Source: CAD feature listing. Evaluate the final solid. Frame: model axes, mm. Face numbers are marked on the shaded views. A direction names the side the tool comes from. Round coordinates to 2 decimals unless told otherwise and drop trailing zeros. Write each loop counter-clockwise with the first axis right and the second up, starting at its lowest first coordinate (ties: lowest second). Pieces come first, ordered by that corner, then holes.
from build123d import *

# Parameters (mm, degrees)
SKETCH1_R                     = 7
BOSS_EXTRUDE1_DEPTH           = 15
BOSS_EXTRUDE1_TAPER           = 3
BOSS_EXTRUDE1_OTHER_WAY_DEPTH = 6
BOSS_EXTRUDE1_OTHER_WAY_TAPER = -3
CUT_EXTRUDE1_DEPTH            = 19.220929184
CUT_EXTRUDE1_DEPTH_BACK       = 19.220929184
CUT_EXTRUDE2_START            = -9.200504543
CUT_EXTRUDE2_OUTLINE_W        = 6.502745185
CUT_EXTRUDE2_OUTLINE_H        = 6
CUT_EXTRUDE2_DEPTH            = 9.200504543
SKETCH5_R                     = 1.5
CUT_EXTRUDE3_DEPTH            = 21.554832283
FILLET1_SIZE                  = 5
CUT_EXTRUDE4_DEPTH            = 19.096992379
CUT_EXTRUDE4_DEPTH_BACK       = 19.096992379
SKETCH6_W                     = 14.909790155
SKETCH6_H                     = 10.479187812
CUT_EXTRUDE5_DEPTH            = 16.143532008


with BuildPart() as part:
    # Sketch1 → Boss-Extrude1 (new body)
    with BuildSketch(Plane(origin=(0, 0, 0), x_dir=(1, 0, 0), z_dir=(0, 1, 0))):
        Circle(SKETCH1_R)
    extrude(amount=BOSS_EXTRUDE1_DEPTH, taper=BOSS_EXTRUDE1_TAPER)

    # Sketch1 → Boss-Extrude1 other way (add)
    with BuildSketch(Plane(origin=(0, 0, 0), x_dir=(1, 0, 0), z_dir=(0, 1, 0))):
        Circle(SKETCH1_R)
    extrude(amount=-BOSS_EXTRUDE1_OTHER_WAY_DEPTH, taper=BOSS_EXTRUDE1_OTHER_WAY_TAPER)

    # Sketch3 → Cut-Extrude1 (cut, two sides: drawn at the far end of the back side and taken through both)
    with BuildSketch(Plane(origin=(0, 0, 0), x_dir=(0, 0, -1), z_dir=(1, 0, 0)).offset(-CUT_EXTRUDE1_DEPTH_BACK)):
        Polygon((-1.886057768, -6), (-1.886057768, 0), (-9.929766736, 8.043708969), (-9.929766736, -6), align=None)
    extrude(amount=CUT_EXTRUDE1_DEPTH + CUT_EXTRUDE1_DEPTH_BACK, mode=Mode.SUBTRACT)

    # Cut-Extrude2: read off the stored shape, not the designer's step
    # Cut-Extrude2 outline → Cut-Extrude2 (cut)
    with BuildSketch(Plane.XY.offset(1.886057768).offset(CUT_EXTRUDE2_START)):
        with Locations((-8.251372593, -3)):
            Rectangle(CUT_EXTRUDE2_OUTLINE_W, CUT_EXTRUDE2_OUTLINE_H)
        with Locations((8.251372593, -3)):
            Rectangle(CUT_EXTRUDE2_OUTLINE_W, CUT_EXTRUDE2_OUTLINE_H)
    extrude(amount=CUT_EXTRUDE2_DEPTH, mode=Mode.SUBTRACT)

    # Sketch5 → Cut-Extrude3 (cut, through all)
    with BuildSketch(Plane(origin=(5, 0, 0), x_dir=(0, 0, -1), z_dir=(1, 0, 0))):
        with Locations((0.613942232, -3.5)):
            Circle(SKETCH5_R)
    extrude(amount=-CUT_EXTRUDE3_DEPTH, mode=Mode.SUBTRACT)

    # Fillet1
    # a fillet whose section is not a circle: 5 mm, written as the material it takes off along each edge
    with BuildSketch(Plane(origin=(17.5, -6, 1.886057768), x_dir=(0, 0, -1), z_dir=(-1, 0, 0))) as fillet1_piece_1:
        with BuildLine():
            Bezier((FILLET1_SIZE, 0), (0, 0), (0, -FILLET1_SIZE), weights=[1, 1.5, 1])
            Line((0, -FILLET1_SIZE), (0, 0))
            Line((0, 0), (FILLET1_SIZE, 0))
        make_face()
    extrude(amount=35, mode=Mode.SUBTRACT)

    # Fillet2
    # a fillet whose section is not a circle: 10, 5 mm, written as the material it takes off along each edge
    with BuildSketch(Plane(origin=(0, 15, 0), x_dir=(1, 0, 0), z_dir=(0, 0, -1))) as fillet2_piece_1:
        with BuildLine():
            Bezier((6.724247047, 9.738320219), (6.213883311, 0), (1.731099374, 0), weights=[1, 0.818181818, 1])
            Line((1.731099374, 0), (6.213883311, 0))
            Line((6.213883311, 0), (6.724247047, 9.738320219))
        make_face()
    revolve(axis=Axis((0, 15, 0), (0, -1, 0)), mode=Mode.SUBTRACT)

    # Sketch6 → Cut-Extrude4 (cut, two sides: drawn at the far end of the back side and taken through both)
    with BuildSketch(Plane(origin=(0, 0, 0), x_dir=(0, 0, -1), z_dir=(1, 0, 0)).offset(-CUT_EXTRUDE4_DEPTH_BACK)):
        with Locations((0.730648031, 10.501273687)):
            Rectangle(SKETCH6_W, SKETCH6_H)
    extrude(amount=CUT_EXTRUDE4_DEPTH + CUT_EXTRUDE4_DEPTH_BACK, mode=Mode.SUBTRACT)

    # Sketch7 → Cut-Extrude5 (cut, through all)
    with BuildSketch(Plane.XZ.offset(6)):
        with BuildLine():
            Line((4, -3.113942232), (4, -3.499048938))
            ThreePointArc((4, -3.499048938), (0, -5.314446676), (-4, -3.499048938))
            Line((-4, -3.499048938), (-4, -3.113942232))
            Line((-4, -3.113942232), (4, -3.113942232))
        make_face()
    extrude(amount=-CUT_EXTRUDE5_DEPTH, mode=Mode.SUBTRACT)


solid = part.part
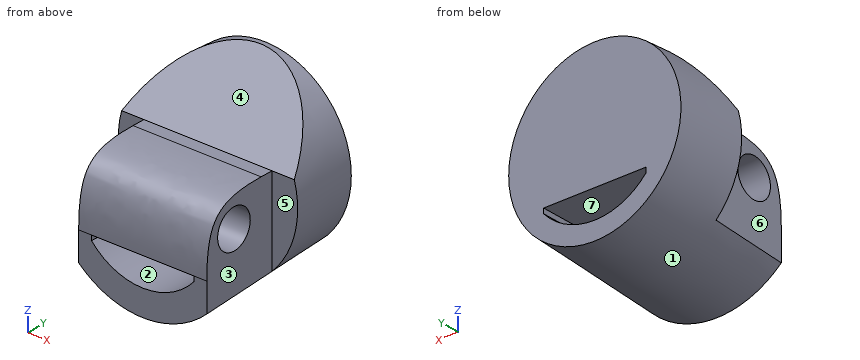
1) Reachability of the marked faces 5, 6 and 7 from +Z, -Z, +X, -X, +Y, -Y: full face, straight path, thin tool, end or side. Return the list, or none.
Taken from the geometry:
face 5: +Z, -Z, +X, -Y
face 6: +Z, -Z, -X, -Y
face 7: +Y, -Y
2) Pull-direction query (X, two-part tool) for the marked faces 1, 2, 3 and 4; classes: released by +X, released by -X, zero draft, split by the parting line, or undercut.
Taken from the geometry:
face 1: split by the parting line
face 2: undercut
face 3: released by +X
face 4: zero draft
3) Section query D-D on y = 0.75. Return the cut outline in (x, z), then the cut area to 3 significant figures.
Taken from the geometry:
outline: (-6.44, 2.64) arc R6.96 ccw (long way) to (6.44, 2.64) - close; hole (-4, -3.5) arc R5.31 ccw to (4, -3.5) - (4, -3.11) - (-4, -3.11) - close
area: 98.8 mm2
4) Section query B-B on y = 4. Return the cut outline in (x, z), then the cut area to 3 significant figures.
Taken from the geometry:
outline: (-3.39, 5.89) arc R6.79 ccw (long way) to (3.39, 5.89) - close; hole (-4, -3.5) arc R5.31 ccw to (4, -3.5) - (4, -3.11) - (-4, -3.11) - close
area: 128 mm2
5) Section query A-A on x = 0. State how many separate pieces and enclosed holes the cut face has, then the cut area to 3 significant figures.
Taken from the geometry:
separate pieces: 2
enclosed holes: 1
area: 79.3 mm2
6) Material intervals for line 1 (Z direction, x = 0, y = -2.75); line 2 (X direction, y = -5, z = 0.25); line 3 (X direction, y = 2.25, z = -4.5), sorted ascending.
Taken from the geometry:
line 1: z = -7.14 to -5.31, -3.11 to -1.91, 0.69 to 1.79
line 2: x = -5 to 5
line 3: x = -5.21 to -2.83, 2.83 to 5.21
7) Contact query for flat-ended pins moving along their axis: P1, Ø3, axis at y = -3, z = 1.5, coming from the +X side; P2, Ø0.6, axis at x = 6, z = -1.5, coming from the -Y side; P3, Ø2, axis at y = -2.5, z = -2, coming from the -X side. Output: stop coordinate, or through.
Taken from the geometry:
P1: stops at x = 5
P2: stops at y = 0
P3: stops at x = -5
